Read the model definition and answer for the solid it produces. Units are mm, in the model's axes. Face numbers are marked on the shaded views. Coordinates: 2 decimals unless noted, no trailing zeros. Write each loop counter-clockwise with the first axis right and the second up, starting at its lowest first coordinate (ties: lowest second). Pieces come first, ordered by that corner, then holes. Notation, with made-up numbers: (2, 26.5) -> (32, 26.5) arc R31 cw to (32, 51.5) -> close; hole circle Ø8 at (4, -10). An arc over 180 degrees is marked (long way). Write item = value, one per line. Start each with the question number.
1) Find the intervals of material crossed by line 1 along Y through (x, z) = (54, 22.86); line 2 along Z through (x, y) = (75.5, 4.5); line 3 along Z through (x, y) = (33, 7), in increasing order. Write a range as from..to.
2) Section C-C (x = 24.5) is taken. Determine the outline of the cut face in (y, z), plus the area to 3 significant figures.
3) Section A-A (z = 22.86) is taken. Determine the outline of the cut face in (x, y), plus the area to 3 significant figures.
4) Section B-B (y = 0) is taken. Determine the outline of the cut face in (x, z), plus the area to 3 significant figures.
5) Section D-D (y = 12) is taken. Determine the outline of the cut face in (x, z).
6) For a pull along Y with two mould halves and no side action, classify the marked faces 1, 2 and 3 as released by +Y, released by -Y, zero draft, split by the parting line, or undercut.
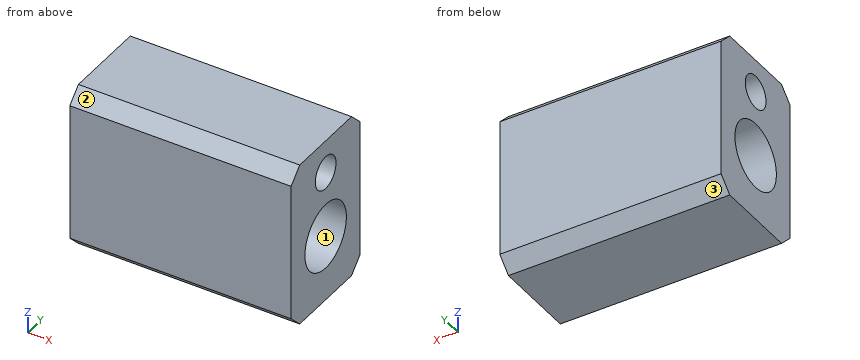
from build123d import *

# Parameters (mm, degrees)
SKETCH1_W           = 50.8
SKETCH1_H           = 76.2
SKETCH1_R           = 15.24
SKETCH1_R_2         = 7.62
BOSS_EXTRUDE1_DEPTH = 101.6
CHAMFER2_SIZE       = 6.35
CHAMFER1_SIZE       = 6.35


with BuildPart() as part:
    # Sketch1 → Boss-Extrude1 (new body)
    with BuildSketch(Plane.YZ):
        Rectangle(SKETCH1_W, SKETCH1_H)
        with Locations(Location((0, -7.62, 0), (0, 0, 270))):
            Circle(SKETCH1_R, mode=Mode.SUBTRACT)
        with Locations(Location((0, 22.86, 0), (0, 0, 270))):
            Circle(SKETCH1_R_2, mode=Mode.SUBTRACT)
    extrude(amount=BOSS_EXTRUDE1_DEPTH)

    # Chamfer2
    chamfer2_edges = [part.edges().sort_by_distance(p)[0] for p in [
        (50.8, -25.4, 38.1),
        (50.8, -25.4, -38.1),
    ]]
    chamfer(chamfer2_edges, length=CHAMFER2_SIZE)

    # Chamfer1
    chamfer1_edges = [part.edges().sort_by_distance(p)[0] for p in [
        (50.8, 25.4, 38.1),
        (50.8, 25.4, -38.1),
    ]]
    chamfer(chamfer1_edges, length=CHAMFER1_SIZE)


solid = part.part
Answer key:
q1.line_1 = -25.4..-7.62, 7.62..25.4
q1.line_2 = -38.1..-22.18, 6.94..16.71, 29.01..38.1
q1.line_3 = -38.1..-21.16, 5.92..19.85, 25.87..38.1
q2.outline = (-25.4, -31.75) -> (-19.05, -38.1) -> (19.05, -38.1) -> (25.4, -31.75) -> (25.4, 31.75) -> (19.05, 38.1) -> (-19.05, 38.1) -> (-25.4, 31.75) -> close; hole circle Ø30.48 at (0, -7.62); hole circle Ø15.24 at (0, 22.86)
q2.area = 2,880 mm^2
q3.outline = (0, -25.4) -> (101.6, -25.4) -> (101.6, -7.62) -> (0, -7.62) -> close; (0, 7.62) -> (101.6, 7.62) -> (101.6, 25.4) -> (0, 25.4) -> close
q3.area = 3,610 mm^2
q4.outline = (0, -38.1) -> (101.6, -38.1) -> (101.6, -22.86) -> (0, -22.86) -> close; (0, 7.62) -> (101.6, 7.62) -> (101.6, 15.24) -> (0, 15.24) -> close; (0, 30.48) -> (101.6, 30.48) -> (101.6, 38.1) -> (0, 38.1) -> close
q4.area = 3,100 mm^2
q5.outline = (0, -38.1) -> (101.6, -38.1) -> (101.6, -17.01) -> (0, -17.01) -> close; (0, 1.77) -> (101.6, 1.77) -> (101.6, 38.1) -> (0, 38.1) -> close
q6.face_1 = undercut
q6.face_2 = released by -Y
q6.face_3 = released by +Y
